```python
from build123d import *

# Parameters (mm, degrees)
SKETCH1_R                      = 130
SKETCH1_R_2                    = 90
BOSS_EXTRUDE1_DEPTH            = 10
SKETCH2_R                      = 7.5
CUT_EXTRUDE1_DEPTH             = 6
CUT_EXTRUDE2_REACH             = 185.946
SKETCH3_R                      = 4
CUT_EXTRUDE2_DIRECTION_2_DEPTH = 184.945644145
CIRPATTERN1_COUNT              = 8


with BuildPart() as part:
    # Sketch1 → Boss-Extrude1 (new body)
    with BuildSketch(Plane(origin=(0, 0, 0), x_dir=(1, 0, 0), z_dir=(0, 1, 0))):
        with Locations(Location((0, 0, 0), (0, 0, 270))):
            Circle(SKETCH1_R)
        with Locations(Location((0, 0, 0), (0, 0, 270))):
            Circle(SKETCH1_R_2, mode=Mode.SUBTRACT)
    extrude(amount=BOSS_EXTRUDE1_DEPTH)

    # Sketch2 → Cut-Extrude1 (cut)
    with BuildSketch(Plane.XZ):
        with Locations(Location((0, 115, 0), (0, 0, 270))):
            Circle(SKETCH2_R)
    cut_extrude1 = extrude(amount=-CUT_EXTRUDE1_DEPTH, mode=Mode.SUBTRACT)

    # Sketch3 → Cut-Extrude2 (cut, up to next)
    with BuildSketch(Plane.XZ.offset(-6), mode=Mode.PRIVATE) as cut_extrude2_sk1:
        with Locations(Location((0, 115, 0), (0, 0, 90))):
            Circle(SKETCH3_R)
    cut_extrude2_tool1 = extrude(cut_extrude2_sk1.sketch, amount=-CUT_EXTRUDE2_REACH, mode=Mode.PRIVATE) & part.part
    cut_extrude2 = cut_extrude2_tool1.solids().sort_by_distance((0, 6, 115))[0]
    add(cut_extrude2, mode=Mode.SUBTRACT)

    # Sketch3 → Cut-Extrude2 direction 2 (cut)
    with BuildSketch(Plane.XZ.offset(-6)):
        with Locations(Location((0, 115, 0), (0, 0, 90))):
            Circle(SKETCH3_R)
    cut_extrude2_direction_2 = extrude(amount=CUT_EXTRUDE2_DIRECTION_2_DEPTH, mode=Mode.SUBTRACT)

    # CirPattern1: Cut-Extrude1, Cut-Extrude2, Cut-Extrude2 direction 2 ×8 about axis
    cirpattern1_axis = Axis((0, 0, 0), (0, 1, 0))
    add([cut_extrude1.rotate(cirpattern1_axis, i * 360 / CIRPATTERN1_COUNT) for i in range(1, CIRPATTERN1_COUNT)], mode=Mode.SUBTRACT)
    add([cut_extrude2.rotate(cirpattern1_axis, i * 360 / CIRPATTERN1_COUNT) for i in range(1, CIRPATTERN1_COUNT)], mode=Mode.SUBTRACT)
    add([cut_extrude2_direction_2.rotate(cirpattern1_axis, i * 360 / CIRPATTERN1_COUNT) for i in range(1, CIRPATTERN1_COUNT)], mode=Mode.SUBTRACT)


solid = part.part
```
Geometry: final body of the model. Coordinates: model frame, mm. A direction names the side the tool comes from. Coordinates: 2 decimals unless noted, no trailing zeros. Order: outer loops, then holes, each group sorted by start corner. A loop starts at its lowest first (then second) coordinate and runs counter-clockwise, first axis right, second up. Notation, with made-up numbers: (8.5, -12) - (17.5, -12) arc R16 cw to (17.5, -8) - close; hole circle Ø9 at (-39.5, -16.5). An arc over 180 degrees is marked (long way). Return JSON: item names as keys, results as strings. Group by question number.
1. Pull-direction query (X, two-part tool) for faces 1 (the face through (87, 0, 28)), 2 (the face through (39.048, 4.93, 123.997)), 3 (the face through (1.532, 7.972, 118.695)); classes: pulls with the +X half, pulls with the -X half, needs draft (parallel to the pull), parting line crosses it, or undercut.
2. Pin query (flat end, axial travel): pin 1 (1 mm diameter, centred on x = -12, y = 4.5, fed in from +Z); pin 2 (1.5 mm diameter, centred on x = 31, y = 8.5, fed in from -Z); pin 3 (16.5 mm diameter, centred on x = -78, z = 80.5, fed in from -Y); pin 4 (2 mm diameter, centred on y = 3, z = -85, fed in from +X). Return the tip coordinate at first contact, or that it passes through.
3. Cut plane B-B (x = 115). Output: boundary loops of the cut face in (y, z), plus the area to 3 significant figures.
4. Cut plane D-D (y = 2.5). Count the separate pieces of the cut face and the enclosed holes in it, plus the area to 3 significant figures.
5. Set-up query: faces 4 (the face through (-107.846, 2.958, 2.253)), 5 (the face through (-83.465, 7.972, -77.943)). Return all of +Z, -Z, +X, -X, +Y, -Y with unobstructed straight access to the full face (end or side cutting, diameter ignored); none if empty.
6. Material intervals for line 1 along Z through (x, y) = (-83, 4.25); line 2 along Z through (x, y) = (4.5, 5); line 3 along X through (y, z) = (3.75, -76.5), sorted ascending. Write a range as [from, to].
7. Cut plane C-C (z = 57). Output: boundary loops of the cut face in (x, y).
8. Cut plane A-A (z = 0). Output: boundary loops of the cut face in (x, y), plus the area to 3 significant figures.
Resolved:
{
 "1": {"face 1": "needs draft", "face 2": "parting line crosses it", "face 3": "undercut"},
 "2": {"pin 1": "stops at z = 129.49", "pin 2": "stops at z = -126.43", "pin 3": "stops at y = 0", "pin 4": "stops at x = 99.22"},
 "3": {"outline": "(0, -60.62) - (10, -60.62) - (10, -4) - (6, -4) - (6, -7.5) - (0, -7.5) - close; (0, 7.5) - (6, 7.5) - (6, 4) - (10, 4) - (10, 60.62) - (0, 60.62) - close", "area": "1,090 mm²"},
 "4": {"separate pieces": "1", "enclosed holes": "9", "area": "26,200 mm²"},
 "5": {"face 4": "-Y", "face 5": "+Y, -Y"},
 "6": {"line 1": "z = [-100.05, -88.63], [-74.01, -34.8], [34.8, 74.01], [88.63, 100.05]", "line 2": "z = [-129.92, -121], [-109, -89.89], [89.89, 109], [121, 129.92]", "line 3": "x = [-105.11, -87.07], [-75.57, -47.41], [47.41, 75.57], [87.07, 105.11]"},
 "7": {"outline": "(-116.84, 0) - (-69.65, 0) - (-69.65, 10) - (-116.84, 10) - close; (69.65, 0) - (116.84, 0) - (116.84, 10) - (69.65, 10) - close"},
 "8": {"outline": "(-130, 0) - (-122.5, 0) - (-122.5, 6) - (-119, 6) - (-119, 10) - (-130, 10) - close; (-111, 6) - (-107.5, 6) - (-107.5, 0) - (-90, 0) - (-90, 10) - (-111, 10) - close; (90, 0) - (107.5, 0) - (107.5, 6) - (111, 6) - (111, 10) - (90, 10) - close; (119, 6) - (122.5, 6) - (122.5, 0) - (130, 0) - (130, 10) - (119, 10) - close", "area": "556 mm²"}
}
